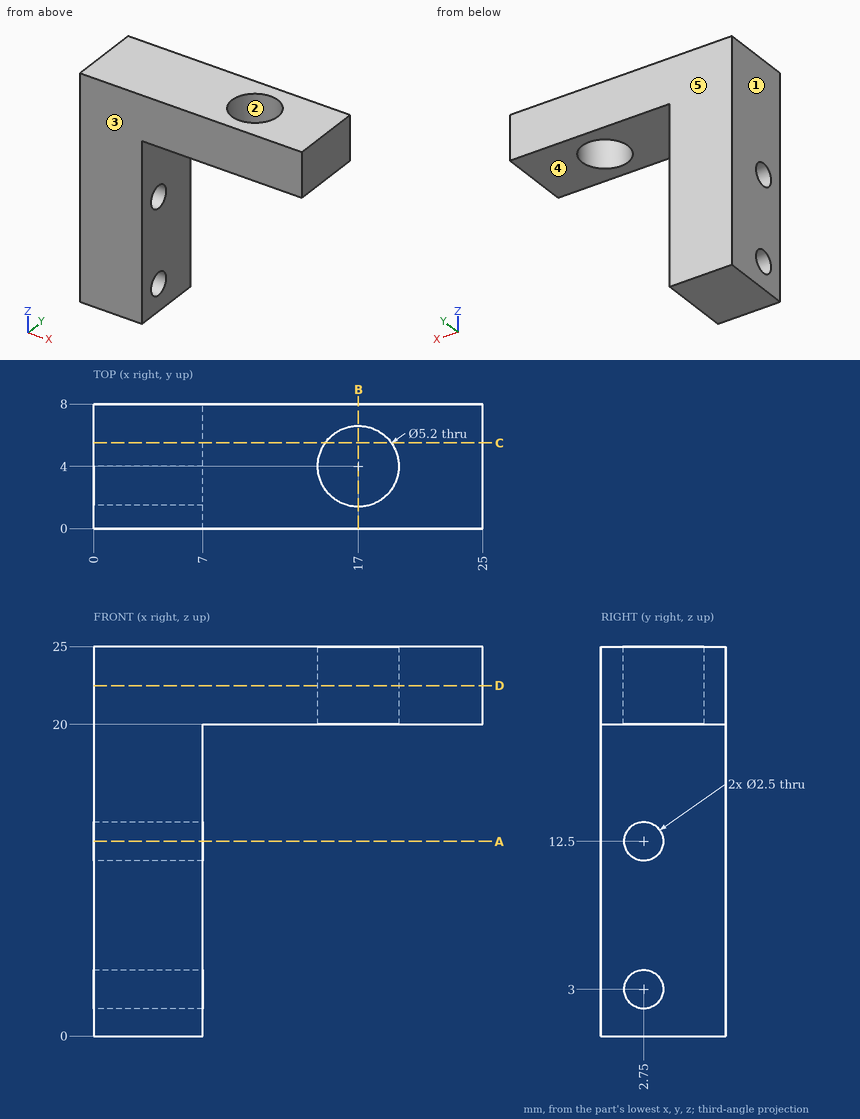
Here's the drawing with two shaded views (mm, measured from the low corner). I have some questions. A direction names the side the tool comes from. Round coordinates to 2 decimals unless told otherwise and drop trailing zeros. Loops run counter-clockwise (first coordinate to the right, second up) from the corner with the lowest first, then second, coordinate; pieces in that order, holes last. Notation, with made-up numbers: M 9,1 L 22,1 A23 ccw 22,28 Z; hole C 1.5,-1 d8. An arc over 180 degrees is marked long. Answer as CSV lines item,"result".
1) Imagine slicing it at C-C on y = 5.5. List the corners of the cut face in (x, z) for me.
From the geometry:
outline,"M 0,0 L 7,0 L 7,20 L 14.88,20 L 14.88,25 L 0,25 Z; M 19.12,20 L 25,20 L 25,25 L 19.12,25 Z"
2) If I drill on probe 1 along Y at (x, z) = (17, 22.55); probe 2 along X at (y, z) = (4.75, 18.5); probe 3 along Z at (x, y) = (9.75, 3.25), over which ranges is the centre line in solid material (lowest first)?
From the geometry:
probe 1,"0 to 1.4, 6.6 to 8"
probe 2,"0 to 7"
probe 3,"20 to 25"
3) For pin 1 Ø4 at (y, z) = (5.5, 11.5) entering from +X, with a flat end and sliding along its axis, tell me the tip position at first contact or that it passes through.
From the geometry:
pin 1,"x = 7"
4) Imagine slicing it at B-B on x = 17. List the corners of the cut face in (y, z) for me, and give its area (3 significant figures).
From the geometry:
outline,"M 0,20 L 1.4,20 L 1.4,25 L 0,25 Z; M 6.6,20 L 8,20 L 8,25 L 6.6,25 Z"
area,"14.0 mm^2"
5) Imagine slicing it at D-D on z = 22.5. List the corners of the cut face in (x, y) for me.
From the geometry:
outline,"M 0,0 L 25,0 L 25,8 L 0,8 Z; hole C 17,4 d5.2"
6) We'd pull the mould along Y, two halves only. Please class the marked faces 1, 2 and 3: released by +Y, released by -Y, zero draft, split by the parting line, or undercut.
From the geometry:
face 1,"zero draft"
face 2,"undercut"
face 3,"released by -Y"
7) Imagine slicing it at A-A on z = 12.5. List the corners of the cut face in (x, y) for me.
From the geometry:
outline,"M 0,0 L 7,0 L 7,1.5 L 0,1.5 Z; M 0,4 L 7,4 L 7,8 L 0,8 Z"
8) Which directions (+Z, -Z, +X, -X, +Y, -Y) give clear straight access to the entire face, cutting with the end or side of a thin tool? Please do the marked faces 4 and 5.
From the geometry:
face 4,"-Z, +X, +Y, -Y"
face 5,"+Z, -Z, +X, -X, +Y"
